Autodesk Inventor part; units mm, degrees
ref_plane "YZ Plane" through (0, 0, 0) normal (1, 0, 0) x (0, 1, 0)
ref_plane "XZ Plane" through (0, 0, 0) normal (0, 1, 0) x (-1, 0, 0)
ref_plane "XY Plane" through (0, 0, 0) normal (0, 0, 1) x (1, 0, 0)
sketch "Sketch1" plane through (0, 0, 0) normal (0, 0, 1) x (1, 0, 0)
  line L0 (1.5, 0) -> (1.5, 40)
  line L1 (3, 0) -> (3, 30)
  line L2 (3, 30) -> (9, 30)
  line L3 (9, 30) -> (9, 40)
  line L4 (9, 40) -> (10.5, 40)
  line L5 (10.5, 40) -> (10.5, 30)
  line L6 (10.5, 30) -> (50.5, 30)
  line L7 (50.5, 30) -> (50.5, 0)
  line L8 (50.5, 0) -> (3, 0)
  point P0 (0, 0)
revolve "Revolution1" add sketch "Sketch1" angle 360 about axis through (1.5, 0, 0) along (0, 1, 0)
sketch "Sketch2" plane through (1.5, 30, 0) normal (0, 1, 0) x (1, 0, 0)
  point P0 (-1.5, 0)
sketch "Sketch4" plane through (1.5, 30, 0) normal (0, 1, 0) x (1, 0, 0)
  circle A0 centre (0, 0) radius 1.5
  circle A1 centre (-10, -25) radius 1
  point P0 (-1.5, 0)
sketch3d "3D Sketch3"
  line L0 (-8.5, 30, 25) -> (-8.5, 34, 25)
  arc A0 (-8.5, 34, 25) -> (-3.5, 39, 25) centre (-3.5, 34, 25) ccw
  line L1 (-3.5, 39, 25) -> (6.5, 39, 25)
  arc A1 (6.5, 39, 25) -> (11.5, 34, 25) centre (6.5, 34, 25) ccw
  line L2 (11.5, 34, 25) -> (11.5, 30, 25)
  dimension "d21" = 5
  dimension "d22" = 5
sweep "Sweep2" add profiles "Sketch4" path "3D Sketch3" contours A1
equation "\"d22\" = d21"
properties part number "bulckhead"
Part model, mm, in its own coordinate system. A direction names the side the tool comes from. Give positions to 0.01 mm unless a question says otherwise; leave off trailing zeros. Loops run counter-clockwise (first coordinate to the right, second up) from the corner with the lowest first, then second, coordinate; pieces in that order, holes last. Notation, with made-up numbers: (45.25, -14.75) -> (94.25, -14.75) arc R11 ccw to (94.25, 2.25) -> close; hole circle Ø8 at (43, -0.75). An arc over 180 degrees is marked (long way). Write each question's results on one line, items separated by ' | '. Start each with the question number.
Q1. Band-saw the part on B-B on z = 0. List the corners of the cut face in (x, y), plus the area to 3 significant figures.
Q2. Band-saw the part on D-D on x = -23. List the corners of the cut face in (y, z).
Q3. Band-saw the part on A-A on x = 1.5. List the corners of the cut face in (y, z), plus the area to 3 significant figures.
Q4. Wall check: L1, parallel to X at y = 8.5, z = 0; L2, parallel to X at y = 32.5, z = 0; L3, parallel to Y at x = -10, z = 14. Give the ranges that are in metal, low to high.
Q5. Pin check, flat tips, straight feed: P1, Ø19.5, axis at x = 1.5, z = 0, coming from the -Y side; P2, Ø5, axis at y = 15, z = -10, coming from the -X side; P3, Ø3, axis at x = -10, z = -4, coming from the +Y side; P4, Ø10, axis at x = 31.5, y = 18, coming from the +Z side. Stop position of each tip, or through.
Q6. Band-saw the part on C-C on y = 8. List the corners of the cut face in (x, z), plus the area to 3 significant figures.
Q7. Pull direction X, two halves, no side cores. Call faces 1 (the face through (-6, 35, 0)), 2 (the face through (-2, 40, -7)), 3 (the face through (1, 30, 2)), 4 (the face through (27.84, 14.79, 41.32)): +X half, -X half, draft (parallel to the pull), parting line (faces both ways), or undercut.
Q8. Which spindle directions (+Z, -Z, +X, -X, +Y, -Y) get a long thin tool onto all of the face, cutting with end or side? Do faces 5 (the face through (0.328, 34.93, 8.923)), 6 (the face through (0.3, 15.2, 0.9)). Say none if no direction does.
Results are:
1) outline: (-47.5, 0) -> (0, 0) -> (0, 30) -> (-6, 30) -> (-6, 40) -> (-7.5, 40) -> (-7.5, 30) -> (-47.5, 30) -> close; (3, 0) -> (50.5, 0) -> (50.5, 30) -> (10.5, 30) -> (10.5, 40) -> (9, 40) -> (9, 30) -> (3, 30) -> close | area: 2,880 mm²
2) outline: (0, -42.44) -> (30, -42.44) -> (30, 42.44) -> (0, 42.44) -> close
3) outline: (0, -49) -> (30, -49) -> (30, -9) -> (40, -9) -> (40, -7.5) -> (30, -7.5) -> (30, -1.5) -> (0, -1.5) -> close; (0, 1.5) -> (30, 1.5) -> (30, 7.5) -> (40, 7.5) -> (40, 9) -> (30, 9) -> (30, 49) -> (0, 49) -> close; circle Ø2 at (39, 25) | area: 2,880 mm²
4) L1: x = -47.5 to 0, 3 to 50.5 | L2: x = -7.5 to -6, 9 to 10.5 | L3: y = 0 to 30
5) P1: stops at y = 0 | P2: stops at x = -46.92 | P3: stops at y = 30 | P4: stops at z = 42.14
6) outline: circle Ø98 at (1.5, 0); hole circle Ø3 at (1.5, 0) | area: 7,540 mm²
7) face 1: undercut | face 2: draft | face 3: undercut | face 4: parting line
8) face 5: +Y | face 6: +Y, -Y
